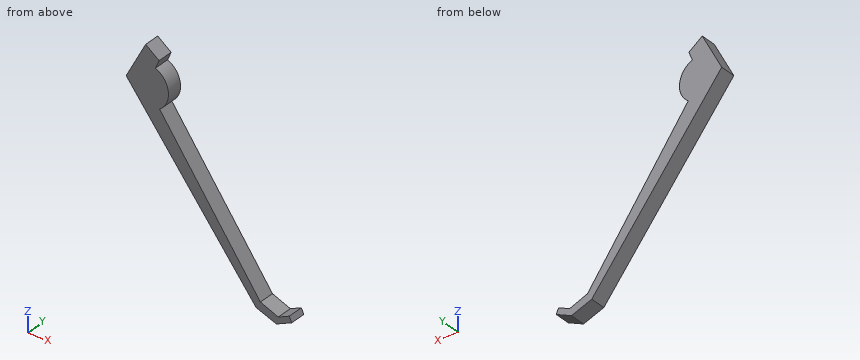
```python
from build123d import *

# Parameters (mm, degrees)
F1_DEPTH = 12.7


with BuildPart() as f1:
    # F0 (on Front) → F1 (new body)
    with BuildSketch(Plane.XZ):
        with BuildLine():
            Line((-32.091238, 46.31887), (-43.157175, 54.539282))
            Line((-43.157175, 54.539282), (-59.281833, 23.870818))
            Line((-59.281833, 23.870818), (48.215881, -112.714514))
            Line((48.215881, -112.714514), (64.972878, -118.721738))
            Line((64.972878, -118.721738), (77.619664, -112.714514))
            Line((77.619664, -112.714514), (75.567222, -108.393584))
            Line((75.567222, -108.393584), (66.470528, -112.714514))
            Line((66.470528, -112.714514), (51.693749, -107.023455))
            Line((51.693749, -107.023455), (-31.634918, 8.961036))
            ThreePointArc((-31.634918, 8.961036), (-24.419928, 25.180798), (-35.020864, 39.420072))
            Line((-35.020864, 39.420072), (-32.091238, 46.31887))
        make_face()
    extrude(amount=F1_DEPTH)


solid = f1.part
```
Model file for the job. Use its own axes, mm. Coordinates: 2 decimals unless noted, no trailing zeros. Write each loop counter-clockwise with the first axis right and the second up, starting at its lowest first coordinate (ties: lowest second). Pieces come first, ordered by that corner, then holes. Notation, with made-up numbers: (65, 51.25) - (84, 51.25) arc R23 ccw to (84, 87.25) - close; hole circle Ø6 at (9, 11.5). An arc over 180 degrees is marked (long way). Use a Markdown table: item, result. Add a question column.
Item 1: Band-saw the part on B-B, the plane x = -22. Write the cut outline in (y, z).
Item 2: Band-saw the part on C-C, the plane z = 3.5. Write the cut outline in (x, y), and give its area (3 significant figures).
Item 3: Drill centre lines: line 1 along Z through (x, y) = (-26, -1.5); line 2 along Z through (x, y) = (-28.5, -11.5); line 3 along Z through (x, y) = (-1, -6.75). Where is each one in solid material? Low to high.
Item 4: Drop flat-ended pins along their axis: pin 1 (3 mm diameter, centred on y = -4, z = -66.5, fed in from -X); pin 2 (4 mm diameter, centred on x = 48.5, y = -9, fed in from +Z); pin 3 (2 mm diameter, centred on y = -9, z = -89.5, fed in from -X). Give the stop position or say it passes through.
Item 5: Band-saw the part on A-A, the plane y = -10.25. Write the cut outline in (x, z), and give its area (3 significant figures).
A:
| question | item | result |
|---|---|---|
| 1 | outline | (-12.7, -23.5) - (0, -23.5) - (0, -4.45) - (-12.7, -4.45) - close |
| 2 | outline | (-43.25, -12.7) - (-27.71, -12.7) - (-27.71, 0) - (-43.25, 0) - close |
| 2 | area | 197 mm² |
| 3 | line 1 | z = -18.42 to 1.12, 15.72 to 30.75 |
| 3 | line 2 | z = -15.24 to 4.6, 11.85 to 34.63 |
| 3 | line 3 | z = -50.18 to -33.68 |
| 4 | pin 1 | stops at x = 10.66 |
| 4 | pin 2 | stops at z = -99.79 |
| 4 | pin 3 | stops at x = 29.16 |
| 5 | outline | (-59.28, 23.87) - (48.22, -112.71) - (64.97, -118.72) - (77.62, -112.71) - (75.57, -108.39) - (66.47, -112.71) - (51.69, -107.02) - (-31.63, 8.96) arc R17.58 ccw to (-35.02, 39.42) - (-32.09, 46.32) - (-43.16, 54.54) - close |
| 5 | area | 2,580 mm² |
